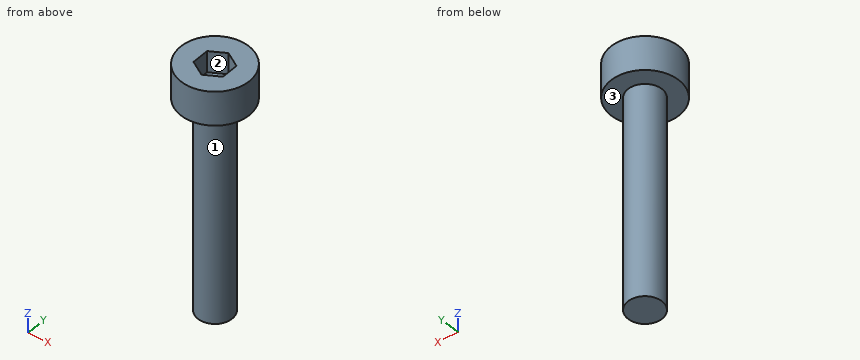
from build123d import *

# Parameters (mm, degrees)
F0_R     = 4
F1_DEPTH = 50
F0_R_2   = 8
F2_DEPTH = 8
F4_DEPTH = 5


with BuildPart() as f1:
    # F0 (on Top) → F1 (new body)
    with BuildSketch(Plane.XY):
        Circle(F0_R)
    extrude(amount=-F1_DEPTH)

    # F0 (on Top) → F2 (join)
    with BuildSketch(Plane.XY):
        Circle(F0_R_2)
        Circle(F0_R, mode=Mode.SUBTRACT)
        Circle(F0_R)
    extrude(amount=F2_DEPTH)

    # F3 (on face) → F4 (cut)
    with BuildSketch(Plane.XY.offset(8)):
        Polygon((-0.012543, 3.953086), (-3.429744, 1.965681), (-3.417202, -1.987405), (0.012543, -3.953086), (3.429744, -1.965681), (3.417202, 1.987405), align=None)
    extrude(amount=-F4_DEPTH, mode=Mode.SUBTRACT)


solid = f1.part
Could you check a few things on this model? Use its own coordinates, in mm. Face numbers are marked on the shaded views. Round coordinates to 2 decimals unless told otherwise and drop trailing zeros. Order: outer loops, then holes, each group sorted by start corner. A loop starts at its lowest first (then second) coordinate and runs counter-clockwise, first axis right, second up.
Q1. Please list where these lines run through material, in increasing order: probe 1 along Z at (x, y) = (5, 0.5); probe 2 along Z at (x, y) = (-1.75, 2.5); probe 3 along X at (y, z) = (-0.25, -34.5).
Geometry says:
probe 1: z = 0 to 8
probe 2: z = -50 to 3
probe 3: x = -3.99 to 3.99
Q2. Thinking about a two-plate mould opening in Y: for the marked faces 1, 2 and 3, which applies, released by +Y, released by -Y, zero draft, split by the parting line, or undercut?
Geometry says:
face 1: split by the parting line
face 2: undercut
face 3: zero draft
Q3. Imagine slicing it at D-D, the plane y = 0. List the corners of the cut face in (x, z) for me, then the cut area to 3 significant figures.
Geometry says:
outline: (-8, 0) - (-4, 0) - (-4, -50) - (4, -50) - (4, 0) - (8, 0) - (8, 8) - (3.42, 8) - (3.42, 3) - (-3.42, 3) - (-3.42, 8) - (-8, 8) - close
area: 494 mm2
Q4. Imagine slicing it at B-B, the plane z = -28.5. List the corners of the cut face in (x, y) for me.
Geometry says:
outline: circle Ø8 at (0, 0)
Q5. Imagine slicing it at A-A, the plane y = -3. List the corners of the cut face in (x, z) for me, then the cut area to 3 significant figures.
Geometry says:
outline: (-7.42, 0) - (-2.65, 0) - (-2.65, -50) - (2.65, -50) - (2.65, 0) - (7.42, 0) - (7.42, 8) - (1.65, 8) - (1.65, 3) - (-1.65, 3) - (-1.65, 8) - (-7.42, 8) - close
area: 367 mm2
Q6. Imagine slicing it at C-C, the plane x = 5. List the corners of the cut face in (y, z) for me (3 decimals), then the cut area to 3 significant figures.
Geometry says:
outline: (-6.245, 0) - (6.245, 0) - (6.245, 8) - (-6.245, 8) - close
area: 99.9 mm2
Q7. I'm going to push flat-ended pins straight in: P1, Ø1.5, axis at x = -1, z = -26.5, coming from the +Y side; P2, Ø1.5, axis at x = -1.5, y = 1.5, coming from the +Z side; P3, Ø1.5, axis at y = 6, z = -25.5, coming from the -X side; P4, Ø1, axis at y = 3.5, z = -2.5, coming from the -X side. Where does each tip first touch, or does it pass through?
Geometry says:
P1: stops at y = 3.99
P2: stops at z = 3
P3: passes through
P4: stops at x = -2.65
